For this review, take the finished solid that the model builds, in its own axes (mm). Face numbers are marked on the shaded views. A direction names the side the tool comes from. Give positions to 0.01 mm unless a question says otherwise; leave off trailing zeros. Write each loop counter-clockwise with the first axis right and the second up, starting at its lowest first coordinate (ties: lowest second). Pieces come first, ordered by that corner, then holes. Notation, with made-up numbers: (17, -28.5) -> (26, -28.5) arc R24 ccw to (26, -13.5) -> close; hole circle Ø7 at (-27, 12.25). An arc over 180 degrees is marked (long way). Write item = value, one per line.
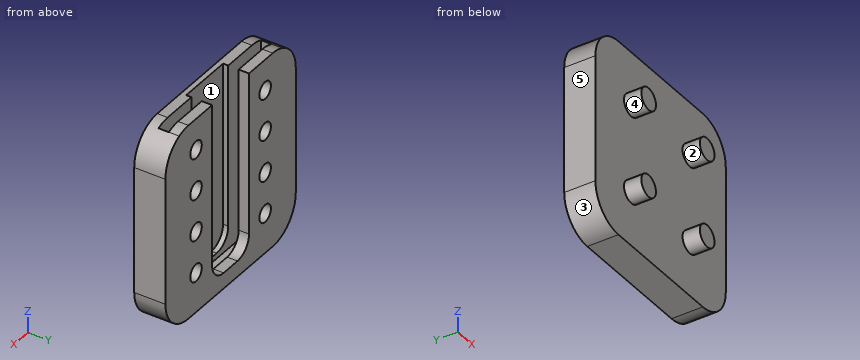
```python
from build123d import *

# Parameters (mm, degrees)
EXTRUDE_1_DEPTH     = 3
SKETCH_3_R          = 3.18
EXTRUDE_2_DEPTH     = 8
EXTRUDE_3_DEPTH     = 3
EXTRUDE_4_DEPTH     = 3
SKETCH_7_R          = 2.5
CUT_EXTRUDE_1_DEPTH = 7.5


with BuildPart() as part:
    # 草图2 → 凸台-拉伸1 (new body)
    with BuildSketch(Plane(origin=(0, 0, 0), x_dir=(1, 0, 0), z_dir=(0, 1, 0))):
        with BuildLine():
            Line((28.284271247, -18.284271247), (28.284271247, 18.284271247))
            ThreePointArc((28.284271247, 18.284271247), (25.355339059, 25.355339059), (18.284271247, 28.284271247))
            Line((18.284271247, 28.284271247), (-18.284271247, 28.284271247))
            ThreePointArc((-18.284271247, 28.284271247), (-25.355339059, 25.355339059), (-28.284271247, 18.284271247))
            Line((-28.284271247, 18.284271247), (-28.284271247, -18.284271247))
            ThreePointArc((-28.284271247, -18.284271247), (-25.355339059, -25.355339059), (-18.284271247, -28.284271247))
            Line((-18.284271247, -28.284271247), (18.284271247, -28.284271247))
            ThreePointArc((18.284271247, -28.284271247), (25.355339059, -25.355339059), (28.284271247, -18.284271247))
        make_face()
    extrude(amount=EXTRUDE_1_DEPTH)

    # 草图3 → 凸台-拉伸2 (add)
    with BuildSketch(Plane(origin=(0, 3, 0), x_dir=(1, 0, 0), z_dir=(0, 1, 0))):
        with Locations(Location((12.7, 12.7, 0), (0, 0, 270))):
            Circle(SKETCH_3_R)
        with Locations(Location((12.7, -12.7, 0), (0, 0, 270))):
            Circle(SKETCH_3_R)
        with Locations(Location((-12.7, -12.7, 0), (0, 0, 270))):
            Circle(SKETCH_3_R)
        with Locations(Location((-12.7, 12.7, 0), (0, 0, 270))):
            Circle(SKETCH_3_R)
    extrude(amount=-EXTRUDE_2_DEPTH)

    # 草图5 → 凸台-拉伸3 (add)
    with BuildSketch(Plane(origin=(0, 3, 0), x_dir=(1, 0, 0), z_dir=(0, 1, 0))):
        with BuildLine():
            Line((-12.284271247, 25.284271247), (12.284271247, 25.284271247))
            ThreePointArc((12.284271247, 25.284271247), (19.355339059, 22.355339059), (22.284271247, 15.284271247))
            Line((22.284271247, 15.284271247), (22.284271247, -27.449422637))
            ThreePointArc((22.284271247, -27.449422637), (26.650871513, -23.761496823), (28.284271247, -18.284271247))
            Line((28.284271247, -18.284271247), (28.284271247, 18.284271247))
            ThreePointArc((28.284271247, 18.284271247), (25.355339059, 25.355339059), (18.284271247, 28.284271247))
            Line((18.284271247, 28.284271247), (-18.284271247, 28.284271247))
            ThreePointArc((-18.284271247, 28.284271247), (-25.355339059, 25.355339059), (-28.284271247, 18.284271247))
            Line((-28.284271247, 18.284271247), (-28.284271247, -18.284271247))
            ThreePointArc((-28.284271247, -18.284271247), (-26.650871513, -23.761496823), (-22.284271247, -27.449422637))
            Line((-22.284271247, -27.449422637), (-22.284271247, 15.284271247))
            ThreePointArc((-22.284271247, 15.284271247), (-19.355339059, 22.355339059), (-12.284271247, 25.284271247))
        make_face()
    extrude(amount=EXTRUDE_3_DEPTH)

    # 草图6 → 凸台-拉伸4 (add)
    with BuildSketch(Plane(origin=(0, 6, 0), x_dir=(1, 0, 0), z_dir=(0, 1, 0))):
        with BuildLine():
            Line((-28.284271247, 18.284271247), (-28.284271247, -18.284271247))
            ThreePointArc((-28.284271247, -18.284271247), (-26.650871513, -23.761496823), (-22.284271247, -27.449422637))
            ThreePointArc((-22.284271247, -27.449422637), (-20.327367684, -28.073334377), (-18.284271247, -28.284271247))
            Line((-18.284271247, -28.284271247), (18.284271247, -28.284271247))
            ThreePointArc((18.284271247, -28.284271247), (20.327367684, -28.073334377), (22.284271247, -27.449422637))
            ThreePointArc((22.284271247, -27.449422637), (26.650871513, -23.761496823), (28.284271247, -18.284271247))
            Line((28.284271247, -18.284271247), (28.284271247, 18.284271247))
            ThreePointArc((28.284271247, 18.284271247), (25.355339059, 25.355339059), (18.284271247, 28.284271247))
            Line((18.284271247, 28.284271247), (-18.284271247, 28.284271247))
            ThreePointArc((-18.284271247, 28.284271247), (-25.355339059, 25.355339059), (-28.284271247, 18.284271247))
        make_face()
    extrude(amount=EXTRUDE_4_DEPTH)

    # 草图7 → 切除-拉伸1 (cut)
    with BuildSketch(Plane(origin=(0, 9, 0), x_dir=(1, 0, 0), z_dir=(0, 1, 0))):
        with Locations(Location((-15, 16.715728753, 0), (0, 0, 270))):
            Circle(SKETCH_7_R)
        with Locations(Location((-15, 4.715728753, 0), (0, 0, 270))):
            Circle(SKETCH_7_R)
        with Locations(Location((-15, -7.284271247, 0), (0, 0, 270))):
            Circle(SKETCH_7_R)
        with Locations(Location((-15, -19.284271247, 0), (0, 0, 270))):
            Circle(SKETCH_7_R)
        with Locations(Location((15, -19.284271247, 0), (0, 0, 270))):
            Circle(SKETCH_7_R)
        with Locations(Location((15, -7.284271247, 0), (0, 0, 270))):
            Circle(SKETCH_7_R)
        with Locations(Location((15, 4.715728753, 0), (0, 0, 270))):
            Circle(SKETCH_7_R)
        with Locations(Location((15, 16.715728753, 0), (0, 0, 270))):
            Circle(SKETCH_7_R)
        with BuildLine():
            Line((-8, -28.284271247), (8, -28.284271247))
            Line((8, -28.284271247), (8, 18.715728753))
            ThreePointArc((8, 18.715728753), (6.535533906, 22.251262658), (3, 23.715728753))
            Line((3, 23.715728753), (-3, 23.715728753))
            ThreePointArc((-3, 23.715728753), (-6.535533906, 22.251262658), (-8, 18.715728753))
            Line((-8, 18.715728753), (-8, -28.284271247))
        make_face()
    extrude(amount=-CUT_EXTRUDE_1_DEPTH, mode=Mode.SUBTRACT)


solid = part.part
```
(1) To check wall thickness, follow probe 1 along Y at (x, z) = (-9.5, -3); probe 2 along X at (y, z) = (3.25, -2); probe 3 along X at (y, z) = (2.25, 12). State the ranges of each line that lie inside material, in increasing order.
Answers below:
probe_1 = 0 to 3, 6 to 9
probe_2 = -28.28 to -22.28, 22.28 to 28.28
probe_3 = -28.28 to -8, 8 to 28.28
(2) The part is to be moulded in two halves that separate along Z. For the marked faces 1, 2 and 3, say which applies: released by +Z, released by -Z, zero draft, split by the parting line, or undercut.
Answers below:
face_1 = zero draft
face_2 = undercut
face_3 = released by -Z
(3) Take a section at B-B (z = -12.7). Write out the cut boundary in (x, y).
Answers below:
outline = (-28.28, 0) -> (-15.88, 0) -> (-15.88, -5) -> (-9.52, -5) -> (-9.52, 0) -> (9.52, 0) -> (9.52, -5) -> (15.88, -5) -> (15.88, 0) -> (28.28, 0) -> (28.28, 9) -> (8, 9) -> (8, 6) -> (22.28, 6) -> (22.28, 3) -> (8, 3) -> (8, 1.5) -> (-8, 1.5) -> (-8, 3) -> (-22.28, 3) -> (-22.28, 6) -> (-8, 6) -> (-8, 9) -> (-28.28, 9) -> close
(4) Take a section at C-C (x = -15). Count the separate pieces of the cut face and the enclosed holes in it, plus the area to 3 significant figures.
Answers below:
separate_pieces = 5
enclosed_holes = 0
area = 303 mm^2
(5) Tool access review of the marked faces 4 and 5: name each direction out of +Z, -Z, +X, -X, +Y, -Y from which nothing blocks a thin tool from reaching the whole face with its end or side.
Answers below:
face_4 = -Y
face_5 = +Z, -Z, -X, +Y, -Y
(6) For pin 1 (4 mm diameter, centred on x = -15, z = 7.28, fed in from +Y); pin 2 (3 mm diameter, centred on x = -18, y = -2, fed in from -Z); pin 3 (3.5 mm diameter, centred on x = 1, y = 7, fed in from +Z); pin 4 (8 mm diameter, centred on x = 15, z = -4.72, fed in from -Y), all flat-tipped, find the tip position at first contact; note any pin that passes through.
Answers below:
pin_1 = 1.5
pin_2 = through
pin_3 = -23.72
pin_4 = 0
(7) Take a section at D-D (x = 21.5). Write out the cut boundary in (y, z).
Answers below:
outline = (0, -27.75) -> (9, -27.75) -> (9, 27.75) -> (6, 27.75) -> (6, -19.17) -> (3, -19.17) -> (3, 27.75) -> (0, 27.75) -> close
(8) Take a section at A-A (y = -2). Write out the cut boundary in (x, z), plus the area to 3 significant figures.
Answers below:
outline = circle Ø6.36 at (-12.7, -12.7); circle Ø6.36 at (-12.7, 12.7); circle Ø6.36 at (12.7, -12.7); circle Ø6.36 at (12.7, 12.7)
area = 127 mm^2
